Input: dimensioned drawing with shaded views. Units: mm. Origin: part minimum x, y, z. A direction names the side the tool comes from. Round coordinates to 2 decimals unless told otherwise and drop trailing zeros. Loops run counter-clockwise (first coordinate to the right, second up) from the corner with the lowest first, then second, coordinate; pieces in that order, holes last.
1) Section B-B, the plane z = 5. Return loops of the section in (x, y).
2) Section C-C, the plane y = 2.2. Return loops of the section in (x, z), and give its area (3 significant figures).
3) Draft query along X for the marked faces 1 and 2. Return one class per face: pulls with the +X half, pulls with the -X half, needs draft (parallel to the pull), parting line crosses it, or undercut.
4) First-contact query: pin 1 (1 mm diameter, centred on y = 1, z = 4, fed in from -X). Flat tip, straight axial feed; report the tip coordinate or a pass-through.
5) Access query for the marked faces 3 and 4. Directions: +Z, -Z, +X, -X, +Y, -Y. A direction counts if a zero-diameter tool reaches every point of the face in a straight line with its end or side. Return the directions, or none.
6) Ray query, line 1 along Z through (x, y) = (5, 3.9); line 2 along Z through (x, y) = (5, 2.45). Return the intervals inside material, ascending.
7) Section A-A, the plane x = 5. Return loops of the section in (y, z).
8) Section D-D, the plane x = 8.5. Return loops of the section in (y, z), and give its area (3 significant figures).
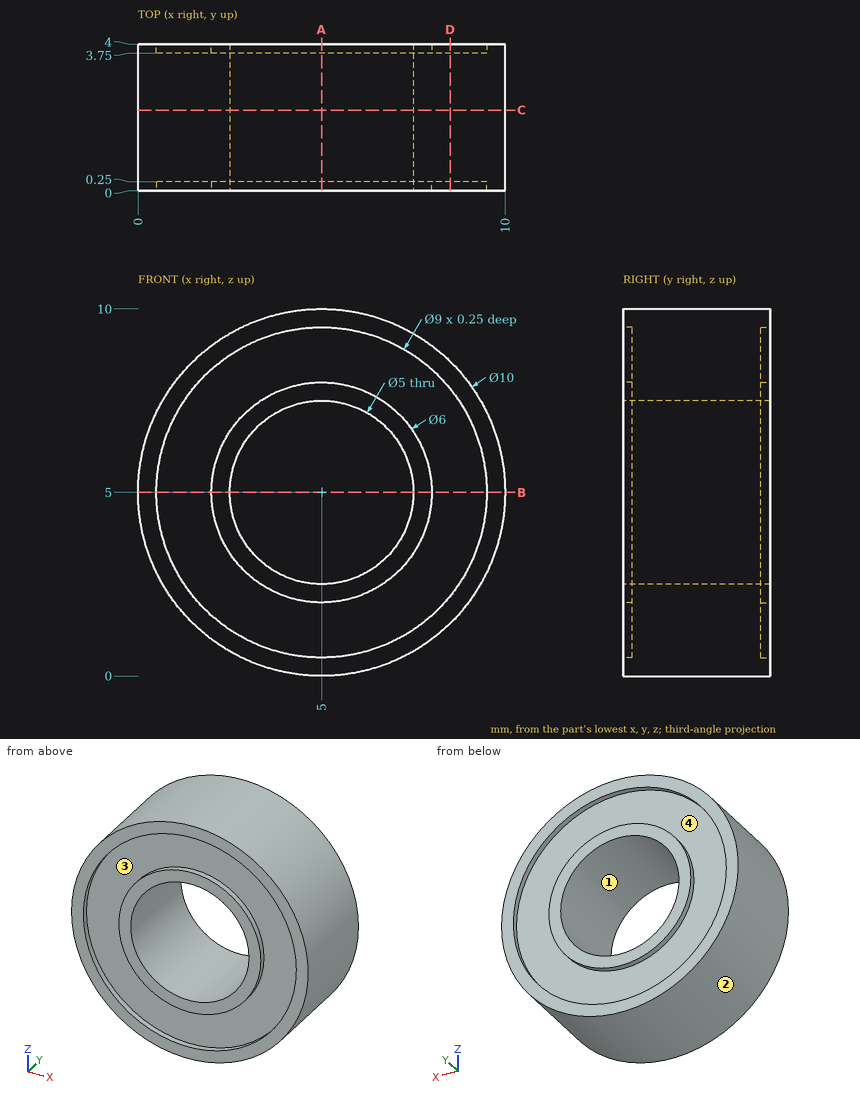
Final values:
1. outline: (0, 0) - (0.5, 0) - (0.5, 0.25) - (2, 0.25) - (2, 0) - (2.5, 0) - (2.5, 4) - (2, 4) - (2, 3.75) - (0.5, 3.75) - (0.5, 4) - (0, 4) - close; (7.5, 0) - (8, 0) - (8, 0.25) - (9.5, 0.25) - (9.5, 0) - (10, 0) - (10, 4) - (9.5, 4) - (9.5, 3.75) - (8, 3.75) - (8, 4) - (7.5, 4) - close
2. outline: circle Ø10 at (5, 5); hole circle Ø5 at (5, 5)
2. area: 58.9 mm2
3. face 1: undercut
3. face 2: parting line crosses it
4. pin 1: stops at x = 0.03
5. face 3: -Y
5. face 4: +Y
6. line 1: z = 0 to 0.5, 2 to 2.5, 7.5 to 8, 9.5 to 10
6. line 2: z = 0 to 2.5, 7.5 to 10
7. outline: (0, 0) - (4, 0) - (4, 0.5) - (3.75, 0.5) - (3.75, 2) - (4, 2) - (4, 2.5) - (0, 2.5) - (0, 2) - (0.25, 2) - (0.25, 0.5) - (0, 0.5) - close; (0, 7.5) - (4, 7.5) - (4, 8) - (3.75, 8) - (3.75, 9.5) - (4, 9.5) - (4, 10) - (0, 10) - (0, 9.5) - (0.25, 9.5) - (0.25, 8) - (0, 8) - close
8. outline: (0, 1.43) - (4, 1.43) - (4, 2.17) - (3.75, 2.17) - (3.75, 7.83) - (4, 7.83) - (4, 8.57) - (0, 8.57) - (0, 7.83) - (0.25, 7.83) - (0.25, 2.17) - (0, 2.17) - close
8. area: 25.7 mm2
